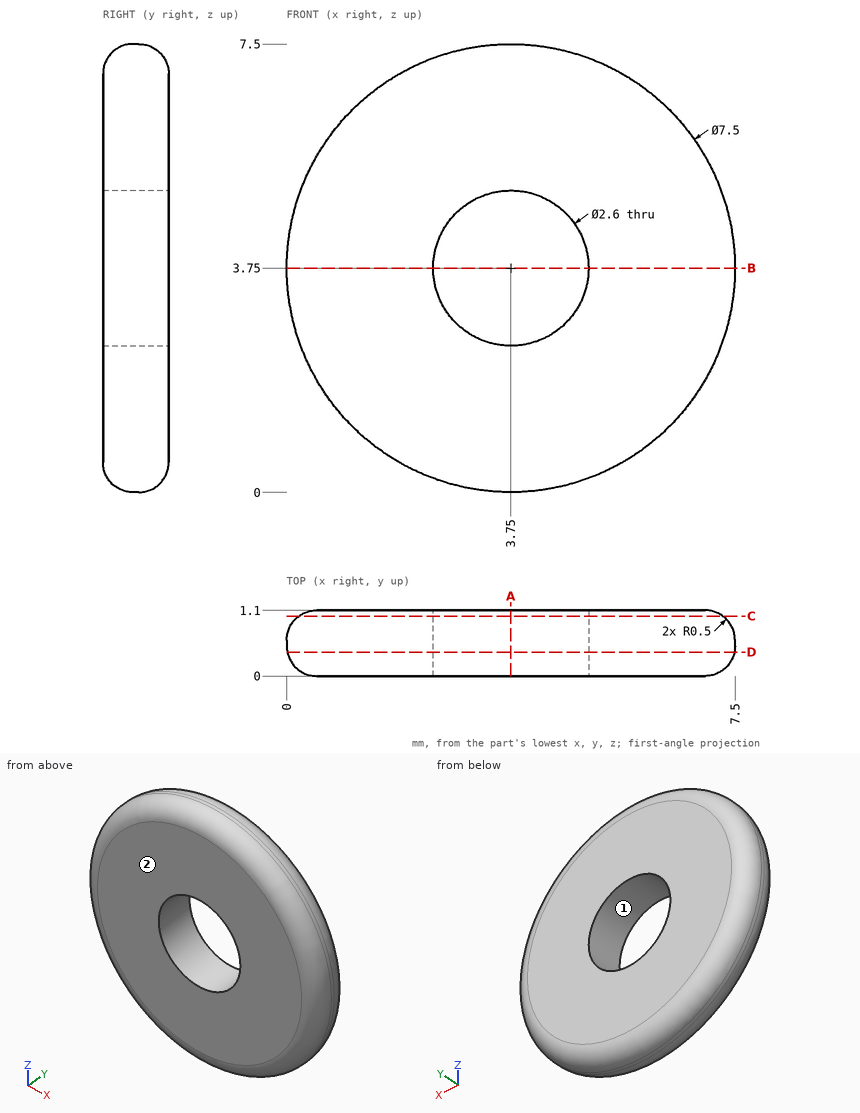
Geometry check sheet. Reference: drawing and pictorial views, mm from the part's lowest x, y, z. Give positions to 0.01 mm unless a question says otherwise; leave off trailing zeros. Write each loop counter-clockwise with the first axis right and the second up, starting at its lowest first coordinate (ties: lowest second). Pieces come first, ordered by that corner, then holes. Notation, with made-up numbers: (53, 21) -> (59, 21) arc R29 cw to (59, 46) -> close; hole circle Ø10 at (70, 45.5). An arc over 180 degrees is marked (long way). One line per item, written item: value. Start each with the question number.
Item 1: Section check B-B on z = 3.75. Record the cut outline in (x, y), then the cut area to 3 significant figures.
Item 2: Section check D-D on y = 0.4. Record the cut outline in (x, z).
Item 3: Material ranges on probe 1 along X at (y, z) = (0.65, 3.75); probe 2 along Z at (x, y) = (3.75, 0.2), recorded low to high. Write a range as from..to.
Item 4: Section check A-A on x = 3.75. Record the cut outline in (y, z).
Item 5: Section check C-C on y = 1. Record the cut outline in (x, z), then the cut area to 3 significant figures.
Item 6: Draft check along X on the marked faces 1 and 2. Enter one of: +X half, -X half, draft (parallel to the pull), parting line (faces both ways), or undercut.
Results list:
1. outline: (0, 0.5) arc R0.5 ccw to (0.5, 0) -> (2.45, 0) -> (2.45, 1.1) -> (0.5, 1.1) arc R0.5 ccw to (0, 0.6) -> close; (5.05, 0) -> (7, 0) arc R0.5 ccw to (7.5, 0.5) -> (7.5, 0.6) arc R0.5 ccw to (7, 1.1) -> (5.05, 1.1) -> close
1. area: 5.18 mm²
2. outline: circle Ø7.48 at (3.75, 3.75); hole circle Ø2.6 at (3.75, 3.75)
3. probe 1: 0..2.45, 5.05..7.5
3. probe 2: 0.1..2.45, 5.05..7.4
4. outline: (0, 0.5) arc R0.5 ccw to (0.5, 0) -> (0.6, 0) arc R0.5 ccw to (1.1, 0.5) -> (1.1, 2.45) -> (0, 2.45) -> close; (0, 5.05) -> (1.1, 5.05) -> (1.1, 7) arc R0.5 ccw to (0.6, 7.5) -> (0.5, 7.5) arc R0.5 ccw to (0, 7) -> close
5. outline: circle Ø7.1 at (3.75, 3.75); hole circle Ø2.6 at (3.75, 3.75)
5. area: 34.3 mm²
6. face 1: undercut
6. face 2: draft
